```python
from build123d import *

# Parameters (mm, degrees)
BOSS_EXTRUDE1_DEPTH = 50
SKETCH3_R           = 17
CUT_EXTRUDE1_DEPTH  = 10
SKETCH4_R           = 2.75
CUT_EXTRUDE2_DEPTH  = 30
FILLET1_R           = 5


with BuildPart() as part:
    # Sketch2 → Boss-Extrude1 (new body)
    with BuildSketch(Plane(origin=(0, 0, 0), x_dir=(0, 0, -1), z_dir=(1, 0, 0))):
        Polygon((0, 0), (0, 50), (-45, 50), (-10, 15), (-10, 0), align=None)
    extrude(amount=BOSS_EXTRUDE1_DEPTH)

    # Sketch3 → Cut-Extrude1 (cut)
    with BuildSketch(Plane.XY.offset(10)):
        with Locations((-4.626643485, -4.843430201)):
            Circle(SKETCH3_R)
    extrude(amount=-CUT_EXTRUDE1_DEPTH, mode=Mode.SUBTRACT)

    # Sketch4 → Cut-Extrude2 (cut)
    with BuildSketch(Plane.XY.offset(10)):
        with Locations((6.441325863, 8.36656836)):
            Circle(SKETCH4_R)
        with Locations((43.550213874, 8.36656836)):
            Circle(SKETCH4_R)
    extrude(amount=-CUT_EXTRUDE2_DEPTH, mode=Mode.SUBTRACT)

    # Fillet1
    fillet1_edges = [part.edges().sort_by_distance(p)[0] for p in [
        (25, 50, 45),
    ]]
    fillet(fillet1_edges, radius=FILLET1_R)


solid = part.part
```
Could you check a few things on this model? Use its own coordinates, in mm. A direction names the side the tool comes from. Round coordinates to 2 decimals unless told otherwise and drop trailing zeros. Write each loop counter-clockwise with the first axis right and the second up, starting at its lowest first coordinate (ties: lowest second). Pieces come first, ordered by that corner, then holes. Notation, with made-up numbers: M 50,-1.75 L 70,-1.75 A22 ccw 70,30.25 Z; hole C 55,-9 d4. An arc over 180 degrees is marked long. Answer in a Markdown table with one row per item. Add a question column.
Q1. If I drill on line 1 (Z direction, x = 33, y = 2); line 2 (Y direction, x = 15.5, z = 13); line 3 (Z direction, x = 7, y = 24.5), over which ranges is the centre line in solid material (lowest first)? Write a range as from..to.
Q2. Imagine slicing it at C-C (z = 11). Please give me the cut outline in (x, y).
Q3. If we mould it in two halves opening along X, with no side actions, what happens to faces 3 (the cylindrical face through (46.09, 7.31, 5.07)), 4 (the flat face through (50, 31, 15)), 5 (the flat face through (0, 35, 15))? For each: +X half, -X half, draft (parallel to the pull), parting line (faces both ways), or undercut.
Q4. Imagine slicing it at D-D (y = 28.5). Please give me the cut outline in (x, z), then the cut area to 4 significant figures.
Q5. On a 3-axis mill with a long thin cutter (end or side, diameter ignored), from which of +Z, -Z, +X, -X, +Y, -Y can I reach the whole of each face in a straight line? I mean faces 1 (the flat face through (30, 8, 10)), 2 (the flat face through (31, 0, 5)). Say none if no direction works.
Q6. Imagine slicing it at B-B (x = 26). Please give me the cut outline in (y, z).
Q7. Imagine slicing it at A-A (x = 42). Please give me the cut outline in (y, z).
Q8. Will these pins go through, and if not, where does the flat tip stop? pin 1 Ø12 at (x, z) = (17.5, 31) entering from -Y; pin 2 Ø6 at (x, z) = (42.5, 32.5) entering from -Y; pin 3 Ø16.5 at (x, y) = (31.5, 8.5) entering from +Z.
Values:
| question | item | result |
|---|---|---|
| 1 | line 1 | 0..10 |
| 1 | line 2 | 18..50 |
| 1 | line 3 | 0..19.5 |
| 2 | outline | M 0,16 L 50,16 L 50,50 L 0,50 Z |
| 3 | face 3 | undercut |
| 3 | face 4 | +X half |
| 3 | face 5 | -X half |
| 4 | outline | M 0,0 L 50,0 L 50,23.5 L 0,23.5 Z |
| 4 | area | 1,175 mm^2 |
| 5 | face 1 | +Z, +X, -X, -Y |
| 5 | face 2 | +Z, -Z, +X, -X, -Y |
| 6 | outline | M 0,0 L 50,0 L 50,32.93 A5 ccw 41.46,36.46 L 15,10 L 0,10 Z |
| 7 | outline | M 0,0 L 6.1,0 L 6.1,10 L 0,10 Z; M 10.64,0 L 50,0 L 50,32.93 A5 ccw 41.46,36.46 L 15,10 L 10.64,10 Z |
| 8 | pin 1 | y = 30 |
| 8 | pin 2 | y = 34.5 |
| 8 | pin 3 | z = 11.75 |
